The listing builds one solid part. Answer for the finished solid, in the listing's coordinates (mm). Face numbers are marked on the shaded views. A direction names the side the tool comes from. Round coordinates to 2 decimals unless told otherwise and drop trailing zeros. Order: outer loops, then holes, each group sorted by start corner. A loop starts at its lowest first (then second) coordinate and runs counter-clockwise, first axis right, second up. Notation, with made-up numbers: (-23, -28) - (15, -28) arc R28 cw to (15, 3) - close; hole circle Ø3 at (17, 55.25). An arc over 180 degrees is marked (long way). One line per item, written item: value. Start each with the question number.
1. Straight lines are drawn through the part: line 1 (Y direction, x = 7.5, z = 9.25) (3 decimals); line 2 (Y direction, x = -11.5, z = 1.25) (3 decimals); line 3 (Z direction, x = -4.5, y = 97.5). For each, find the intervals that lie inside material, in ascending order.
2. For a pull along Y with two mould halves and no side action, classify the marked faces 1, 2, 3 and 4 as released by +Y, released by -Y, zero draft, split by the parting line, or undercut.
3. A tool of negligible diameter and unlimited length cuts with its end or side. For the marked faces 5 and 6, from which of +Z, -Z, +X, -X, +Y, -Y can it reach the whole face along a straight path? Write none if from no direction.
4. Section C-C, the plane y = 101 is taken. Give the vertices of the cut face in (x, z), then the cut area to 3 significant figures.
5. Section A-A, the plane x = -3.5 is taken. Give the vertices of the cut face in (y, z) (3 decimals), then the cut area to 3 significant figures.
6. Section B-B, the plane x = 14 is taken. Give the vertices of the cut face in (y, z).
7. Flat-ended cylindrical pins translate along their axes: P1, Ø1.9, axis at y = 123.5, z = 6.5, coming from the +X side; P2, Ø6, axis at y = 92, z = 2, coming from the -X side; P3, Ø1.9, axis at x = 5.5, z = 6.5, coming from the +Y side (3 decimals). Find the tip coordinate at first contact, or state that the pin passes through.
8. Section D-D, the plane y = 66 is taken. Give the vertices of the cut face in (x, z).
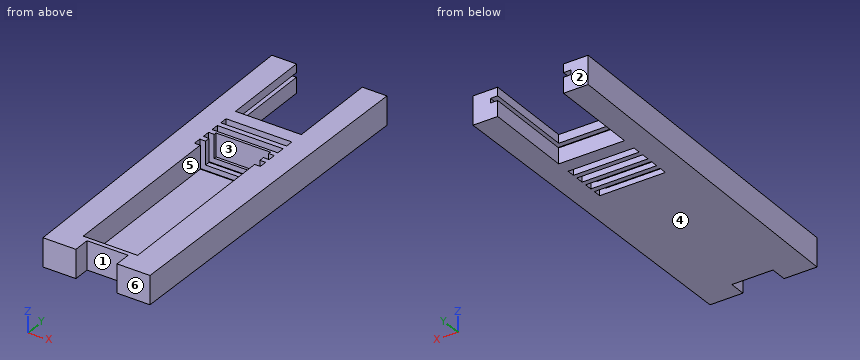
from build123d import *

# Parameters (mm, degrees)
PAD_DEPTH       = 11
SKETCH001_W     = 25.4
SKETCH001_H     = 3
POCKET_DEPTH    = 11.001
SKETCH003_W     = 31
SKETCH003_H     = 1.75
POCKET001_DEPTH = 37
SKETCH004_W     = 21
SKETCH004_H     = 76
POCKET002_DEPTH = 9


with BuildPart() as part:
    # Sketch → Pad (new body)
    with BuildSketch(Plane.XY):
        Polygon((-22.225, 133.35), (-20.6375, 0), (-7.9375, 0), (-7.9375, 6.35), (7.9375, 6.35), (7.9375, 0), (20.6375, 0), (22.225, 133.35), (12.7, 133.35), (12.7, 98.425), (-12.7, 98.425), (-12.7, 133.35), align=None)
    extrude(amount=PAD_DEPTH)

    # Sketch001 → Pocket (cut, through all)
    with BuildSketch(Plane.XY.offset(11)):
        with Locations((0, 91.5)):
            Rectangle(SKETCH001_W, SKETCH001_H)
        with Locations((0, 86.5)):
            Rectangle(SKETCH001_W, SKETCH001_H)
        with Locations((0, 81.5)):
            Rectangle(SKETCH001_W, SKETCH001_H)
        with Locations((0, 76.5)):
            Rectangle(SKETCH001_W, SKETCH001_H)
    extrude(amount=-POCKET_DEPTH, mode=Mode.SUBTRACT)

    # Sketch003 → Pocket001 (cut)
    with BuildSketch(Plane(origin=(0, 133.35, 0), x_dir=(-1, 0, 0), z_dir=(0, 1, 0))):
        with Locations((0, 6.875)):
            Rectangle(SKETCH003_W, SKETCH003_H)
    extrude(amount=-POCKET001_DEPTH, mode=Mode.SUBTRACT)

    # Sketch004 → Pocket002 (cut)
    with BuildSketch(Plane.XY.offset(11)):
        with Locations((0, 46)):
            Rectangle(SKETCH004_W, SKETCH004_H)
    extrude(amount=-POCKET002_DEPTH, mode=Mode.SUBTRACT)


solid = part.part
Answer list:
1. line 1: y = 6.35 to 8, 84 to 85, 88 to 90, 93 to 98.425
1. line 2: y = 0 to 75, 78 to 80, 83 to 85, 88 to 90, 93 to 98.425
1. line 3: z = 0 to 6, 7.75 to 11
2. face 1: released by -Y
2. face 2: released by +Y
2. face 3: undercut
2. face 4: zero draft
3. face 5: +Z
3. face 6: +Z, -Z, +X, -X, -Y
4. outline: (-21.84, 0) - (-12.7, 0) - (-12.7, 6) - (-15.5, 6) - (-15.5, 7.75) - (-12.7, 7.75) - (-12.7, 11) - (-21.84, 11) - close; (12.7, 0) - (21.84, 0) - (21.84, 11) - (12.7, 11) - (12.7, 7.75) - (15.5, 7.75) - (15.5, 6) - (12.7, 6) - close
4. area: 191 mm²
5. outline: (6.35, 0) - (75, 0) - (75, 2) - (8, 2) - (8, 11) - (6.35, 11) - close; (78, 0) - (80, 0) - (80, 2) - (78, 2) - close; (83, 0) - (85, 0) - (85, 11) - (84, 11) - (84, 2) - (83, 2) - close; (88, 0) - (90, 0) - (90, 11) - (88, 11) - close; (93, 0) - (98.425, 0) - (98.425, 6) - (96.35, 6) - (96.35, 7.75) - (98.425, 7.75) - (98.425, 11) - (93, 11) - close
5. area: 247 mm²
6. outline: (0, 0) - (133.35, 0) - (133.35, 6) - (96.35, 6) - (96.35, 7.75) - (133.35, 7.75) - (133.35, 11) - (0, 11) - close
7. P1: stops at x = 22.12
7. P2: stops at x = -21.77
7. P3: stops at y = 98.425
8. outline: (-21.42, 0) - (21.42, 0) - (21.42, 11) - (10.5, 11) - (10.5, 2) - (-10.5, 2) - (-10.5, 11) - (-21.42, 11) - close
